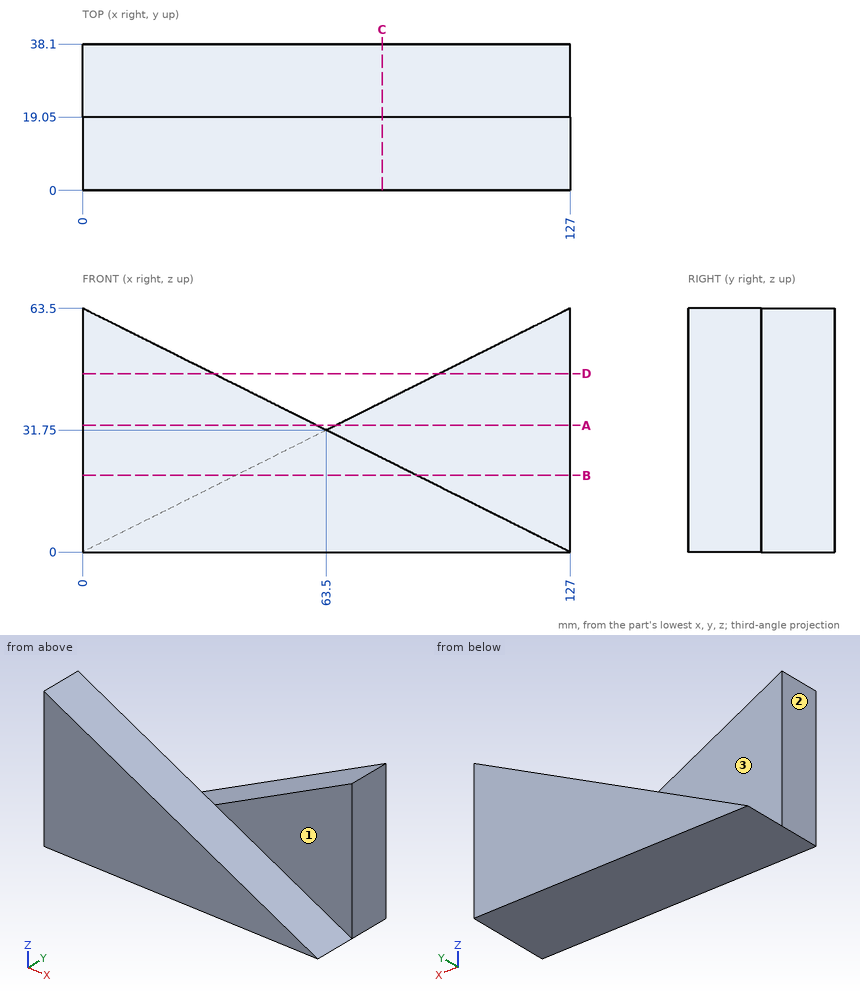
The figure shows three views and two pictorial views of one solid part (mm, origin at its lowest corner). Answer the questions. A direction names the side the tool comes from. Give positions to 0.01 mm unless a question says otherwise; leave off trailing zeros. Write each loop counter-clockwise with the first axis right and the second up, starting at its lowest first coordinate (ties: lowest second). Pieces come first, ordered by that corner, then holes. Notation, with made-up numbers: (41, -10.75) -> (82, -10.75) arc R20 cw to (82, 26.25) -> close; hole circle Ø4 at (21, 53). An arc over 180 degrees is marked (long way). Answer as a JSON object with one key per item and string values.
1) Section C-C on x = 78 is taken. Write down the section's boundary in (y, z), then the cut area to 3 significant figures.
Findings below:
{"outline": "(0, 0) -> (38.1, 0) -> (38.1, 39) -> (19.05, 39) -> (19.05, 24.5) -> (0, 24.5) -> close", "area": "1,210 mm^2"}
2) Section B-B on z = 20 is taken. Write down the section's boundary in (x, y), then the cut area to 3 significant figures.
Findings below:
{"outline": "(0, 0) -> (87, 0) -> (87, 19.05) -> (127, 19.05) -> (127, 38.1) -> (40, 38.1) -> (40, 19.05) -> (0, 19.05) -> close", "area": "3,310 mm^2"}
3) A tool of negligible diameter and unlimited length cuts with its end or side. For the marked faces 1, 2 and 3, from which of +Z, -Z, +X, -X, +Y, -Y can it reach the whole face along a straight path? Write none if from no direction.
Findings below:
{"face 1": "+Z, +X, -Y", "face 2": "+Z, -Z, -X, +Y, -Y", "face 3": "+Z, -X, +Y"}
4) Straight lines are drawn through the part: probe 1 along Y at (x, z) = (119, 23); probe 2 along Y at (x, z) = (13, 27); probe 3 along Z at (x, y) = (104, 22). For each, find the intervals that lie inside material, in ascending order. Write a range as from..to.
Findings below:
{"probe 1": "y = 19.05..38.1", "probe 2": "y = 0..19.05", "probe 3": "z = 0..52"}
5) Section A-A on z = 33 is taken. Write down the section's boundary in (x, y).
Findings below:
{"outline": "(0, 0) -> (61, 0) -> (61, 19.05) -> (0, 19.05) -> close; (66, 19.05) -> (127, 19.05) -> (127, 38.1) -> (66, 38.1) -> close"}
6) Section D-D on z = 46.5 is taken. Write down the section's boundary in (x, y), then the cut area to 3 significant figures.
Findings below:
{"outline": "(0, 0) -> (34, 0) -> (34, 19.05) -> (0, 19.05) -> close; (93, 19.05) -> (127, 19.05) -> (127, 38.1) -> (93, 38.1) -> close", "area": "1,300 mm^2"}
7) Flat-ended cylindrical pins translate along their axes: pin 1 Ø10 at (x, y) = (69.5, 25) entering from +Z; pin 2 Ø3 at (y, z) = (28, 23.5) entering from -X; pin 3 Ø2 at (y, z) = (26.5, 39) entering from -X. Find the tip coordinate at first contact, or state that the pin passes through.
Findings below:
{"pin 1": "stops at z = 37.25", "pin 2": "stops at x = 44", "pin 3": "stops at x = 76"}
